from build123d import *

# Parameters (mm, degrees)
SKETCH1_R           = 2
BOSS_EXTRUDE1_DEPTH = 3


with BuildPart() as part:
    # Sketch1 → Boss-Extrude1 (new body)
    with BuildSketch(Plane(origin=(0, 0, 0), x_dir=(1, 0, 0), z_dir=(0, 1, 0))):
        Polygon((-19, 35), (-40, 10.5), (-45, 10.5), (-45, 5.5), (-40, 5.5), (-40, -2), (-45, -2), (-45, -12), (-40, -12), (-40, -19.5), (-45, -19.5), (-45, -29.5), (-40, -29.5), (-40, -37), (-45, -37), (-45, -44.5), (-40, -44.5), (40, -44.5), (45, -44.5), (45, -37), (40, -37), (40, -29.5), (45, -29.5), (45, -19.5), (40, -19.5), (40, -12), (45, -12), (45, -2), (40, -2), (40, 5.5), (45, 5.5), (45, 10.5), (40, 10.5), (19, 35), align=None)
        with Locations(Location((-36, -12, 0), (0, 0, 270))):
            Circle(SKETCH1_R, mode=Mode.SUBTRACT)
        with Locations(Location((36, -12, 0), (0, 0, 270))):
            Circle(SKETCH1_R, mode=Mode.SUBTRACT)
        with Locations(Location((0, 30, 0), (0, 0, 270))):
            Circle(SKETCH1_R, mode=Mode.SUBTRACT)
    extrude(amount=BOSS_EXTRUDE1_DEPTH)


solid = part.part
Verification items for the finished model (mm, model axes). A direction names the side the tool comes from. Coordinates: 2 decimals unless noted, no trailing zeros. Order: outer loops, then holes, each group sorted by start corner. A loop starts at its lowest first (then second) coordinate and runs counter-clockwise, first axis right, second up. Notation, with made-up numbers: M 26,53.5 L 60,53.5 A13 ccw 60,58.5 Z; hole C 87.25,-34.75 d7. An arc over 180 degrees is marked long. Write each question's results on one line, items separated by ' | '.
1) Release check for a two-part mould opening along Z. For faces 5 (the face through (-45, 1, 41)), 6 (the face through (-40, 1, 33)), 7 (the face through (-29.353, 1.479, -22.922)) record: pulls with the +Z half, pulls with the -Z half, needs draft (parallel to the pull), parting line crosses it, or undercut.
Solved:
face 5: needs draft | face 6: undercut | face 7: pulls with the -Z half
2) Section check C-C on y = 1.6. Give the number of separate pieces and of enclosed holes in the cut face, plus the area to 3 significant figures.
Solved:
separate pieces: 1 | enclosed holes: 3 | area: 6,130 mm²
3) Section check D-D on z = -30. Record the cut outline in (x, y).
Solved:
outline: M -23.29,0 L -2,0 L -2,3 L -23.29,3 Z; M 2,0 L 23.29,0 L 23.29,3 L 2,3 Z
4) Access from +Z, -Z, +X, -X, +Y, -Y to the whole of each face (thin tool, end or side, straight path). Record for faces 1 (the face through (-40, 1, -2)), 2 (the face through (-1, 3, 4)), 3 (the face through (42, 1, 12)), 4 (the face through (-42, 1, -10.5)).
Solved:
face 1: -X, +Y, -Y | face 2: +Z, -Z, +X, -X, +Y | face 3: +X, +Y, -Y | face 4: -Z, -X, +Y, -Y
5) Section check A-A on x = 36. Record the cut outline in (y, z), plus the area to 3 significant figures.
Solved:
outline: M 0,-15.17 L 3,-15.17 L 3,10 L 0,10 Z; M 0,14 L 3,14 L 3,44.5 L 0,44.5 Z | area: 167 mm²
6) Gauge pin test, flat ends, axial feed: pin 1 Ø0.9 at (y, z) = (2, 33.5) entering from -X; pin 2 Ø0.9 at (x, y) = (43, 1.5) entering from -Z; pin 3 Ø0.9 at (y, z) = (2, 35) entering from +X. Record the tip position at first contact, or that the pin passes through.
Solved:
pin 1: stops at x = -40 | pin 2: stops at z = -10.5 | pin 3: stops at x = 40
7) Scan lines: line 1 along X through (y, z) = (2.8, 0); line 2 along X through (y, z) = (2, -30); line 3 along X through (y, z) = (2, 12.5). Record each from-to range of solid material in increasing order. Write a range as [from, to].
Solved:
line 1: x = [-40, 40] | line 2: x = [-23.29, -2], [2, 23.29] | line 3: x = [-40, -37.94], [-34.06, 34.06], [37.94, 40]
8) Section check B-B on z = 11. Record the cut outline in (x, y), plus the area to 3 significant figures.
Solved:
outline: M -45,0 L -37.73,0 L -37.73,3 L -45,3 Z; M -34.27,0 L 34.27,0 L 34.27,3 L -34.27,3 Z; M 37.73,0 L 45,0 L 45,3 L 37.73,3 Z | area: 249 mm²
